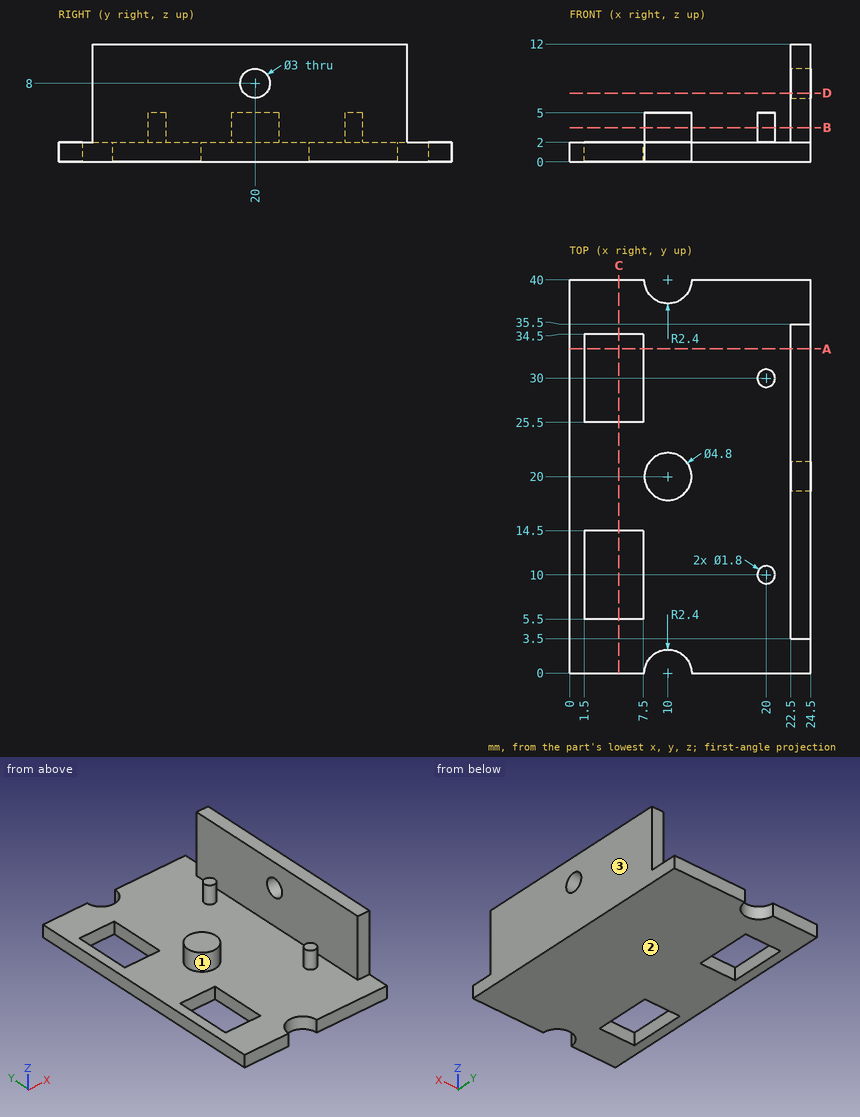
The figure shows three views and two pictorial views of one solid part (mm, origin at its lowest corner). Answer the questions. Coordinates: 2 decimals unless noted, no trailing zeros. Loops run counter-clockwise (first coordinate to the right, second up) from the corner with the lowest first, then second, coordinate; pieces in that order, holes last. Notation, with made-up numbers: (59, 35.5) - (101, 35.5) arc R31 ccw to (101, 71.5) - close; hole circle Ø3 at (48, 68). An arc over 180 degrees is marked (long way). Write item = value, one per line.
1) Section A-A (y = 33) is taken. Determine the outline of the cut face in (x, z).
Responses:
outline = (0, 0) - (1.5, 0) - (1.5, 2) - (0, 2) - close; (7.5, 0) - (24.5, 0) - (24.5, 12) - (22.5, 12) - (22.5, 2) - (7.5, 2) - close
2) Determine the mould class of the marked faces 1, 2 and 3 for opening direction X: pulls with the +X half, pulls with the -X half, needs draft (parallel to the pull), parting line crosses it, or undercut.
Responses:
face_1 = undercut
face_2 = needs draft
face_3 = pulls with the +X half
3) Section B-B (z = 3.5) is taken. Determine the outline of the cut face in (x, y), plus the area to 3 significant figures.
Responses:
outline = circle Ø4.8 at (10, 20); circle Ø1.8 at (20, 10); circle Ø1.8 at (20, 30); (22.5, 3.5) - (24.5, 3.5) - (24.5, 35.5) - (22.5, 35.5) - close
area = 87.2 mm^2
4) Section D-D (z = 7) is taken. Determine the outline of the cut face in (x, y).
Responses:
outline = (22.5, 3.5) - (24.5, 3.5) - (24.5, 18.88) - (22.5, 18.88) - close; (22.5, 21.12) - (24.5, 21.12) - (24.5, 35.5) - (22.5, 35.5) - close
5) Section C-C (x = 5) is taken. Determine the outline of the cut face in (y, z), plus the area to 3 significant figures.
Responses:
outline = (0, 0) - (5.5, 0) - (5.5, 2) - (0, 2) - close; (14.5, 0) - (25.5, 0) - (25.5, 2) - (14.5, 2) - close; (34.5, 0) - (40, 0) - (40, 2) - (34.5, 2) - close
area = 44.0 mm^2
6) Find the intervals of material crossed by line 1 along Z through (x, y) = (23.7, 20); line 2 along Y through (x, z) = (24, 8); line 3 along X through (y, z) = (5.5, 3.75), in increasing order.
Responses:
line_1 = 0 to 6.5, 9.5 to 12
line_2 = 3.5 to 18.5, 21.5 to 35.5
line_3 = 22.5 to 24.5
7) Each of these flat-tipped pins is pushed along its axis until it touches: P1, Ø5, axis at y = 20, z = 8, coming from the -X side; P2, Ø4, axis at x = 21, z = 5.5, coming from the -Y side; P3, Ø2, axis at x = 19.5, y = 10, coming from the +Z side. Where does it stop, or does it pass through?
Responses:
P1 = 22.5
P2 = 3.5
P3 = 5
